```python
from build123d import *

# Parameters (mm, degrees)
SKETCH1_W                       = 287.9979
SKETCH1_H                       = 201.6125
BOSS_EXTRUDE1_DEPTH             = 9.525
FILLET2_R                       = 25.4
F_1_4_CLEARANCE_HOLE1_D         = 6.7564
F_1_4_CLEARANCE_HOLE1_DEPTH     = 21.59
F_1_4_CLEARANCE_HOLE1_TIP       = 2.029827343
F_5_16_CLEARANCE_HOLE1_D        = 8.4328
F_1_4_0_25_DIAMETER_HOLE2_D     = 6.35
F_1_4_0_25_DIAMETER_HOLE2_DEPTH = 21.59
F_1_4_0_25_DIAMETER_HOLE2_TIP   = 1.907732465


with BuildPart() as part:
    # Sketch1 → Boss-Extrude1 (new body)
    with BuildSketch(Plane(origin=(0, 0, 0), x_dir=(1, 0, 0), z_dir=(0, 1, 0))):
        Rectangle(SKETCH1_W, SKETCH1_H)
    extrude(amount=BOSS_EXTRUDE1_DEPTH)

    # Fillet2
    fillet2_edges = [part.edges().sort_by_distance(p)[0] for p in [
        (143.99895, 4.7625, 100.80625),
        (-143.99895, 4.7625, 100.80625),
        (-143.99895, 4.7625, -100.80625),
        (143.99895, 4.7625, -100.80625),
    ]]
    fillet(fillet2_edges, radius=FILLET2_R)

    # 1/4 Clearance Hole1
    with Locations(Plane(origin=(0, 9.525, 0), x_dir=(1, 0, 0), z_dir=(0, 1, 0))):
        with Locations((-131.29895, 75.40625), (131.29895, 75.40625), (131.29895, -76.99375), (-131.29895, -76.99375)):
            Hole(F_1_4_CLEARANCE_HOLE1_D / 2, depth=F_1_4_CLEARANCE_HOLE1_DEPTH)
            with Locations((0, 0, -(F_1_4_CLEARANCE_HOLE1_DEPTH + F_1_4_CLEARANCE_HOLE1_TIP / 2))):  # 118° drill point
                Cone(0, F_1_4_CLEARANCE_HOLE1_D / 2, F_1_4_CLEARANCE_HOLE1_TIP, mode=Mode.SUBTRACT)

    # 5/16 Clearance Hole1 (through all)
    with Locations(Plane(origin=(0, 0, 0), x_dir=(-1, 0, 0), z_dir=(0, -1, 0))):
        with Locations((76.2, -88.10625), (76.2, -65.88125), (42.857421778, 88.10625), (109.542578222, 62.70625), (42.857421778, 62.70625), (109.542578222, 88.10625)):
            Hole(F_5_16_CLEARANCE_HOLE1_D / 2)

    # 1/4 (0.25) Diameter Hole2
    with Locations(Plane(origin=(0, 9.525, 0), x_dir=(1, 0, 0), z_dir=(0, 1, 0))):
        with Locations((53.975, -35.71875), (98.425, -35.71875), (98.425, -61.9125), (98.425, -88.10625), (53.975, -88.10625), (53.975, -61.9125), (-66.675, -7.14375), (-85.725, -7.14375)):
            Hole(F_1_4_0_25_DIAMETER_HOLE2_D / 2, depth=F_1_4_0_25_DIAMETER_HOLE2_DEPTH)
            with Locations((0, 0, -(F_1_4_0_25_DIAMETER_HOLE2_DEPTH + F_1_4_0_25_DIAMETER_HOLE2_TIP / 2))):  # 118° drill point
                Cone(0, F_1_4_0_25_DIAMETER_HOLE2_D / 2, F_1_4_0_25_DIAMETER_HOLE2_TIP, mode=Mode.SUBTRACT)


solid = part.part
```
Model file for the job. Use its own axes, mm. Coordinates: 2 decimals unless noted, no trailing zeros. Order: outer loops, then holes, each group sorted by start corner. A loop starts at its lowest first (then second) coordinate and runs counter-clockwise, first axis right, second up. Notation, with made-up numbers: (5, 64) -> (34, 64) arc R22 cw to (34, 72) -> close; hole circle Ø7 at (59.5, 60.5). An arc over 180 degrees is marked (long way). Return JSON: item names as keys, results as strings.
Item 1: Slice it at B-B (y = 3). Count the separate pieces of the cut face and the enclosed holes in it, then the cut area to 3 significant figures.
Model answer:
{"separate pieces": "1", "enclosed holes": "18", "area": "56,800 mm²"}
Item 2: Mould opens along X. For faces 1 (the face through (54.663, 4.696, 91.206)), 2 (the face through (136.361, 4.829, 93.563)), 3 (the face through (54.663, 4.696, 65.012)), 4 (the face through (-2, 9.525, -1)) say: pulls with the +X half, pulls with the -X half, needs draft (parallel to the pull), parting line crosses it, or undercut.
Model answer:
{"face 1": "undercut", "face 2": "pulls with the +X half", "face 3": "undercut", "face 4": "needs draft"}
Item 3: Wall check: line 1 along Z through (x, y) = (-76.2, 2.5); line 2 along X through (y, z) = (3.75, -73); line 3 along Z through (x, y) = (-43.5, 2). Give the ranges that are in metal, low to high. Write a range as from..to.
Model answer:
{"line 1": "z = -100.81..61.66, 70.1..83.89, 92.32..100.81", "line 2": "x = -144..-133.67, -128.93..128.93, 133.67..144", "line 3": "z = -100.81..-92.27, -83.94..-66.87, -58.54..100.81"}
Item 4: Slice it at A-A (x = -76.2). Write the cut outline in (y, z) (3 decimals), then the cut area to 3 significant figures.
Model answer:
{"outline": "(0, -100.806) -> (9.525, -100.806) -> (9.525, 61.665) -> (0, 61.665) -> close; (0, 70.098) -> (9.525, 70.098) -> (9.525, 83.89) -> (0, 83.89) -> close; (0, 92.323) -> (9.525, 92.323) -> (9.525, 100.806) -> (0, 100.806) -> close", "area": "1,760 mm²"}
Item 5: Pin check, flat tip, straight feed: P1, Ø10, axis at x = 98.42, z = 61.91, coming from the +Y side (3 decimals). Stop position of the tip, or through.
Model answer:
{"P1": "stops at y = 9.525"}
